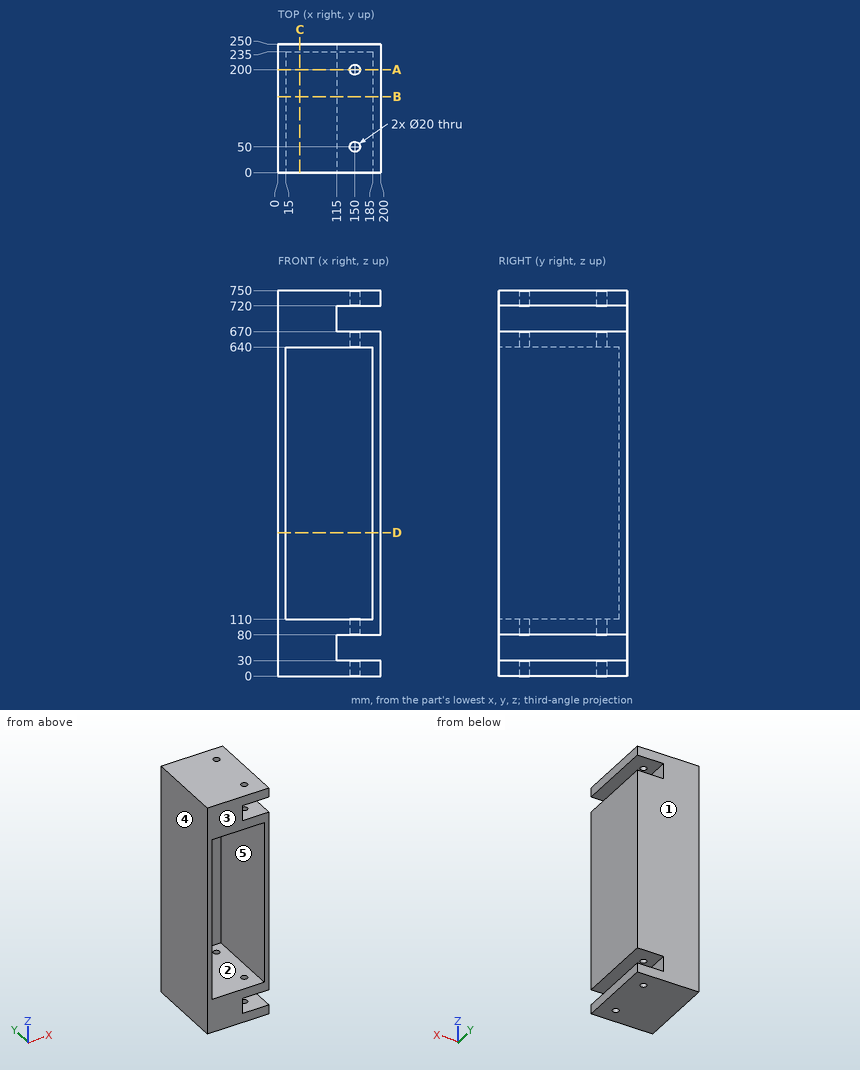
Study the drawing (mm; zero at the part's minimum x, y, z) and answer. A direction names the side the tool comes from. Give positions to 0.01 mm unless a question says otherwise; leave off trailing zeros. Loops run counter-clockwise (first coordinate to the right, second up) from the corner with the lowest first, then second, coordinate; pieces in that order, holes last. Notation, with made-up numbers: (-9.5, 74) -> (37.5, 74) arc R21 cw to (37.5, 85) -> close; hole circle Ø2 at (-27.75, 71). An arc over 180 degrees is marked (long way). Write item = value, one per line. Start each with the question number.
(1) Find section D-D on z = 279. Give the vertices of the cut face in (x, y), and give its area (4 significant figures).
(2) Which of the six approach directions +Z, -Z, +X, -X, +Y, -Y give full straight-line access (tool end or side, diameter ignored) to the marked faces 1 and 2?
(3) Find section B-B on y = 147.5. Give the vertices of the cut face in (x, z), and give its area (3 significant figures).
(4) Find section C-C on x = 43. Give the vertices of the cut face in (y, z), and give its area (4 significant figures).
(5) Given pin 1 Ø18 at (x, y) = (150, 50) entering from -Z; pin 2 Ø8 at (y, z) = (86, 408) entering from -X; pin 3 Ø2 at (y, z) = (66.5, 673) entering from +X; pin 4 Ø10 at (x, z) = (74, 163) entering from -Y, each flat-ended and moving along its own axis, determine where each tip first touches the part or whether it passes through.
(6) The mould has two halves that part along X. Classify the marked faces 3, 4 and 5: +X half, -X half, draft (parallel to the pull), parting line (faces both ways), or undercut.
(7) Find the intervals of material crossed by probe 1 along Y at (x, z) = (150, 97.75); probe 2 along Z at (x, y) = (177.5, 44); probe 3 along X at (y, z) = (59.5, 528.5), in increasing order. Write a range as from..to.
(8) Find section A-A on y = 200. Give the number of separate pieces and of enclosed holes in the cut face, and give its area (3 significant figures).
From the geometry:
q1.outline = (0, 0) -> (15, 0) -> (15, 235) -> (185, 235) -> (185, 0) -> (200, 0) -> (200, 250) -> (0, 250) -> close
q1.area = 10,050 mm^2
q2.face_1 = +Z, -Z, +X, -X, +Y
q2.face_2 = -Y
q3.outline = (0, 0) -> (200, 0) -> (200, 30) -> (115, 30) -> (115, 80) -> (200, 80) -> (200, 670) -> (115, 670) -> (115, 720) -> (200, 720) -> (200, 750) -> (0, 750) -> close; hole (15, 110) -> (185, 110) -> (185, 640) -> (15, 640) -> close
q3.area = 51,400 mm^2
q4.outline = (0, 0) -> (250, 0) -> (250, 750) -> (0, 750) -> (0, 640) -> (235, 640) -> (235, 110) -> (0, 110) -> close
q4.area = 62,950 mm^2
q5.pin_1 = through
q5.pin_2 = 0
q5.pin_3 = 115
q5.pin_4 = 235
q6.face_3 = draft
q6.face_4 = -X half
q6.face_5 = undercut
q7.probe_1 = 0..40, 60..190, 210..250
q7.probe_2 = 0..30, 80..110, 640..670, 720..750
q7.probe_3 = 0..15, 185..200
q8.separate_pieces = 4
q8.enclosed_holes = 0
q8.area = 49,000 mm^2
